Autodesk Inventor part; units mm, degrees
ref_plane "YZ Plane" through (0, 0, 0) normal (1, 0, 0) x (0, 1, 0)
ref_plane "XZ Plane" through (0, 0, 0) normal (0, 1, 0) x (-1, 0, 0)
ref_plane "XY Plane" through (0, 0, 0) normal (0, 0, 1) x (1, 0, 0)
sketch "Sketch1" plane through (0, 0, 0) normal (0, 0, 1) x (1, 0, 0)
  line L0 (0, 0) -> (200, 0)
  line L1 (200, 0) -> (200, -300)
  line L2 (200, -300) -> (1000, -300)
  line L3 (1000, -300) -> (1000, -400)
  line L4 (1000, -400) -> (950, -400)
  line L5 (950, -400) -> (950, -350)
  line L6 (950, -350) -> (50, -350)
  line L7 (50, -350) -> (50, -400)
  line L8 (0, -400) -> (50, -400)
  line L9 (950, -400) -> (1000, -400)
  line L10 (0, -300) -> (100, -300)
  line L11 (100, -300) -> (100, -50)
  line L12 (100, -50) -> (0, -50)
  line L13 (0, 0) -> (0, -50)
  line L14 (0, -300) -> (0, -400)
  dimension "d0" = 200
  dimension "d1" = 300
  dimension "d2" = 800
  dimension "d3" = 100
  dimension "d41" = 50
  dimension "d42" = 900
  dimension "d43" = 100
  dimension "d44" = 250
extrude "Extrusion1" add sketch "Sketch1" along normal blind 250
sketch "Sketch2" plane through (0, 0, 0) normal (0, 1, 0) x (1, 0, 0)
  line L0 (200, 0) -> (0, 0)
  line L1 (200, 0) -> (150, 0)
  line L2 (200, -250) -> (0, -250)
  line L3 (200, -250) -> (150, -250)
  circle A0 centre (165, -50) radius 15
  circle A1 centre (165, -200) radius 15
  line L4 (200, 0) -> (200, -250)
  dimension "d9" = 50
  dimension "d11" = 30
  dimension "d12" = 30
  dimension "d36" = 35
  dimension "d37" = 35
  dimension "d49" = 150
sketch "Sketch4" plane through (0, 0, 0) normal (0, 1, 0) x (1, 0, 0)
  line L0 (200, 0) -> (200, -250)
  line L1 (200, -125) -> (192.5, -125)
  circle A0 centre (192.5, -125) radius 7.5
  point P0 (0, 0)
  dimension "d38" = 7.5
extrude "Extrusion7" add sketch "Sketch4" along normal blind 10
extrude "Extrusion8" cut sketch "Sketch2" against normal blind 30
sketch "Sketch6" plane through (0, 0, 250) normal (0, 0, 1) x (1, 0, 0)
  line L0 (100, -50) -> (100, -300)
  line L1 (100, -300) -> (0, -300)
  line L2 (0, -300) -> (0, -400)
  line L3 (0, -400) -> (50, -400)
  line L4 (50, -400) -> (50, -350)
  line L5 (50, -350) -> (950, -350)
  line L6 (950, -350) -> (950, -400)
  line L7 (950, -400) -> (1000, -400)
  line L8 (1000, -400) -> (1000, -300)
  line L9 (1000, -300) -> (200, -300)
  line L10 (200, -300) -> (200, 0)
  line L11 (200, 0) -> (0, 0)
  line L12 (0, 0) -> (0, -50)
  line L13 (0, -50) -> (100, -50)
  line L14 (200, -400) -> (200, -320)
  line L15 (200, -400) -> (215.7164, -400)
  line L16 (215.7164, -400) -> (915.7164, -400)
  line L17 (915.7164, -400) -> (915.7164, -330)
  circle A0 centre (915.7164, -330) radius 10.5844
  line L18 (200, 0) -> (150, 0)
  line L19 (200, 0) -> (0, 0)
  line L20 (150, 0) -> (150, -20)
  circle A1 centre (150, -20) radius 3
  dimension "d40" = 0
  dimension "d50" = 80
  dimension "d51" = 700
  dimension "d52" = 70
  dimension "d53" = 50
  dimension "d54" = 20
  dimension "d55" = 6
hole "Hole2" at (150, -20, 250) direction (0, 0, -1) diameter 9 depth 20
hole "Hole3" at (200, -320, 250) direction (0, 0, -1) diameter 9 depth 20
properties part number "Platform" material "Wood (Walnut)"
CAD build for the part. Positions are in the model's coordinates, mm. A direction names the side the tool comes from. Coordinates: 2 decimals unless noted, no trailing zeros. Loops run counter-clockwise (first coordinate to the right, second up) from the corner with the lowest first, then second, coordinate; pieces in that order, holes last. Notation, with made-up numbers: (51.25, -5.5) - (70.25, -5.5) arc R14 cw to (70.25, 16.5) - close; hole circle Ø2 at (12, 38.25). An arc over 180 degrees is marked (long way). Use CSV: the item, a comma, the result in double quotes. Start each with the question number.
Q1. Cut at A-A, the plane y = -360. List the corners of the cut face in (x, z).
Q2. 3-axis set-ups, long thin cutter, end or side, ignore diameter. For faces 5 (the flat face through (49, -300, 123)), 6 (the flat face through (0, -25, 123)), 7 (the flat face through (506, -350, 123)), 8 (the flat face through (594, -300, 123)), 9 (the flat face through (165, -30, 200)): which of +Z, -Z, +X, -X, +Y, -Y reach the whole face in a straight line?
Q3. Two-plate mould, pull along Z, no slides. Class faces 1 (the cylindrical face through (153, -15, 209)), 2 (the flat face through (165, -30, 50)), 3 (the flat face through (387, -303, 250)), 4 (the flat face through (975, -400, 123)): +Z half, -Z half, draft (parallel to the pull), parting line (faces both ways), or undercut.
Q4. Cut at C-C, the plane x = 165. List the corners of the cut face in (y, z), then the cut area to 3 significant figures.
Q5. Cut at D-D, the plane y = -135. List the corners of the cut face in (x, z), then the cut area to 3 significant figures.
Q6. Cut at B-B, the plane z = 50. List the corners of the cut face in (x, y).
Q7. Drop flat-ended pins along their axis: P1, Ø1.5, axis at y = -196, z = 100, coming from the -X side; P2, Ø12, axis at x = 508, z = 96.5, coming from the +Y side; P3, Ø24, axis at x = 167.5, z = 43, coming from the +Y side. Give the stop position or say it passes through.
Q8. Probe probe 1 along Z at (x, y) = (165, -7); probe 2 along X at (y, z) = (-320, 237); probe 3 along X at (y, z) = (-361, 180). List the from-to ranges inside material, lowest first. Write a range as from..to.
Here are the results:
1,outline,"(0, 0) - (50, 0) - (50, 250) - (0, 250) - close; (950, 0) - (1000, 0) - (1000, 250) - (950, 250) - close"
2,face 5,"+Z, -Z, -X"
2,face 6,"+Z, -Z, -X, +Y, -Y"
2,face 7,"+Z, -Z, -Y"
2,face 8,"+Z, -Z, +X, +Y"
2,face 9,"+Y"
3,face 1,"undercut"
3,face 2,"undercut"
3,face 3,"+Z half"
3,face 4,"draft"
4,outline,"(-350, 0) - (0, 0) - (0, 35) - (-30, 35) - (-30, 65) - (0, 65) - (0, 185) - (-30, 185) - (-30, 215) - (0, 215) - (0, 250) - (-350, 250) - close"
4,area,"85,700 mm2"
5,outline,"(100, 0) - (200, 0) - (200, 250) - (100, 250) - close"
5,area,"25,000 mm2"
6,outline,"(0, -400) - (50, -400) - (50, -350) - (950, -350) - (950, -400) - (1000, -400) - (1000, -300) - (200, -300) - (200, 0) - (180, 0) - (180, -30) - (150, -30) - (150, 0) - (0, 0) - (0, -50) - (100, -50) - (100, -300) - (0, -300) - close"
7,P1,"x = 100"
7,P2,"y = -300"
7,P3,"y = 0"
8,probe 1,"0..35, 65..185, 215..250"
8,probe 2,"0..195.5, 204.5..1000"
8,probe 3,"0..50, 950..1000"
